```python
from build123d import *

# Parameters (mm, degrees)
F0_W     = 4.2
F0_H     = 4.5
F1_DEPTH = 12
F2_R     = 0.8
F3_SIZE  = 0.5


with BuildPart() as f1:
    # F0 (on Top) → F1 (new body)
    with BuildSketch(Plane.XY):
        Polygon((6, -23.5), (6, 23.5), (2.1, 23.5), (2.1, 19), (-2.1, 19), (-2.1, 23.5), (-6, 23.5), (-6, -23.5), align=None)
        with Locations((0, 21.25)):
            Rectangle(F0_W, F0_H)
        with Locations((0, 25.75)):
            Rectangle(F0_W, F0_H)
    extrude(amount=F1_DEPTH)

    # F2
    f2_edges = [f1.edges().sort_by_distance(p)[0] for p in [
        (2.1, 28, 6),
        (-2.1, 28, 6),
        (6, -23.5, 6),
        (-6, -23.5, 6),
    ]]
    fillet(f2_edges, radius=F2_R)

    # F3
    f3_edges = [f1.edges().sort_by_distance(p)[0] for p in [
        (6, 0.4, 12),
        (5.765685, -23.265685, 12),
        (4.05, 23.5, 12),
        (0, -23.5, 12),
        (2.1, 25.35, 12),
        (-5.765685, -23.265685, 12),
        (1.865685, 27.765685, 12),
        (-6, 0.4, 12),
        (0, 28, 12),
        (-4.05, 23.5, 12),
        (-1.865685, 27.765685, 12),
        (-2.1, 25.35, 12),
        (6, 0.4, 0),
        (5.765685, -23.265685, 0),
        (4.05, 23.5, 0),
        (0, -23.5, 0),
        (2.1, 25.35, 0),
        (-5.765685, -23.265685, 0),
        (1.865685, 27.765685, 0),
        (-6, 0.4, 0),
        (0, 28, 0),
        (-4.05, 23.5, 0),
        (-1.865685, 27.765685, 0),
        (-2.1, 25.35, 0),
    ]]
    chamfer(f3_edges, length=F3_SIZE)


solid = f1.part
```
Could you check a few things on this model? Use its own coordinates, in mm. A direction names the side the tool comes from. Coordinates: 2 decimals unless noted, no trailing zeros. Write each loop counter-clockwise with the first axis right and the second up, starting at its lowest first coordinate (ties: lowest second). Pieces come first, ordered by that corner, then holes. Notation, with made-up numbers: (-31.75, 69) -> (18.25, 69) arc R18 cw to (18.25, 104) -> close; hole circle Ø4 at (86.5, 39). An arc over 180 degrees is marked (long way). Write item = value, one per line. Start each with the question number.
(1) Will these pins go through, and if not, where does the flat tip stop? pin 1 (1 mm diameter, centred on x = -3.5, z = 9.5, fed in from +Y); pin 2 (4.5 mm diameter, centred on x = -3, z = 8, fed in from +Y); pin 3 (1.8 mm diameter, centred on y = 26, z = 6.5, fed in from -X); pin 4 (4.5 mm diameter, centred on x = 4, z = 7, fed in from +Y).
(2) I need wall thicknesses on line 1 (Y direction, x = 3.5, z = 9.5); line 2 (Y direction, x = -5.5, z = 1.25). Which ranges of each line are inside material? Lowest first, please. Write a range as [from, to].
(3) Which directions (+Z, -Z, +X, -X, +Y, -Y) give clear straight access to the entire face, cutting with the end or side of a thin tool? Please do faces 1 (the face through (0, 3, 12)), 2 (the face through (4, 23.5, 6)), 3 (the face through (-4, 23.5, 6)).
(4) I want a section at B-B (z = 6). Please give me the cut outline in (x, y).
(5) I want a section at A-A (x = -3.5). Please give me the cut outline in (y, z).
Result set:
q1.pin_1 = 23.5
q1.pin_2 = 28
q1.pin_3 = -2.1
q1.pin_4 = 27.86
q2.line_1 = [-23.5, 23.5]
q2.line_2 = [-23.44, 23.5]
q3.face_1 = +Z, +X, -X, +Y, -Y
q3.face_2 = +Z, -Z, +X, +Y
q3.face_3 = +Z, -Z, -X, +Y
q4.outline = (-6, -22.7) arc R0.8 ccw to (-5.2, -23.5) -> (5.2, -23.5) arc R0.8 ccw to (6, -22.7) -> (6, 23.5) -> (2.1, 23.5) -> (2.1, 27.2) arc R0.8 ccw to (1.3, 28) -> (-1.3, 28) arc R0.8 ccw to (-2.1, 27.2) -> (-2.1, 23.5) -> (-6, 23.5) -> close
q5.outline = (-23.5, 0.5) -> (-23, 0) -> (23, 0) -> (23.5, 0.5) -> (23.5, 11.5) -> (23, 12) -> (-23, 12) -> (-23.5, 11.5) -> close
